The drawing under review shows one solid part. Ordinate dimensions are in mm from its lowest x, y, z. A direction names the side the tool comes from. Give positions to 0.01 mm unless a question says otherwise; leave off trailing zeros. Loops run counter-clockwise (first coordinate to the right, second up) from the corner with the lowest first, then second, coordinate; pieces in that order, holes last. Notation, with made-up numbers: M 22,20 L 78,20 A22 cw 78,55 Z; hole C 65.5,-20.5 d1. An arc over 180 degrees is marked long. Put each result on its own line as item: value. Start each with the question number.
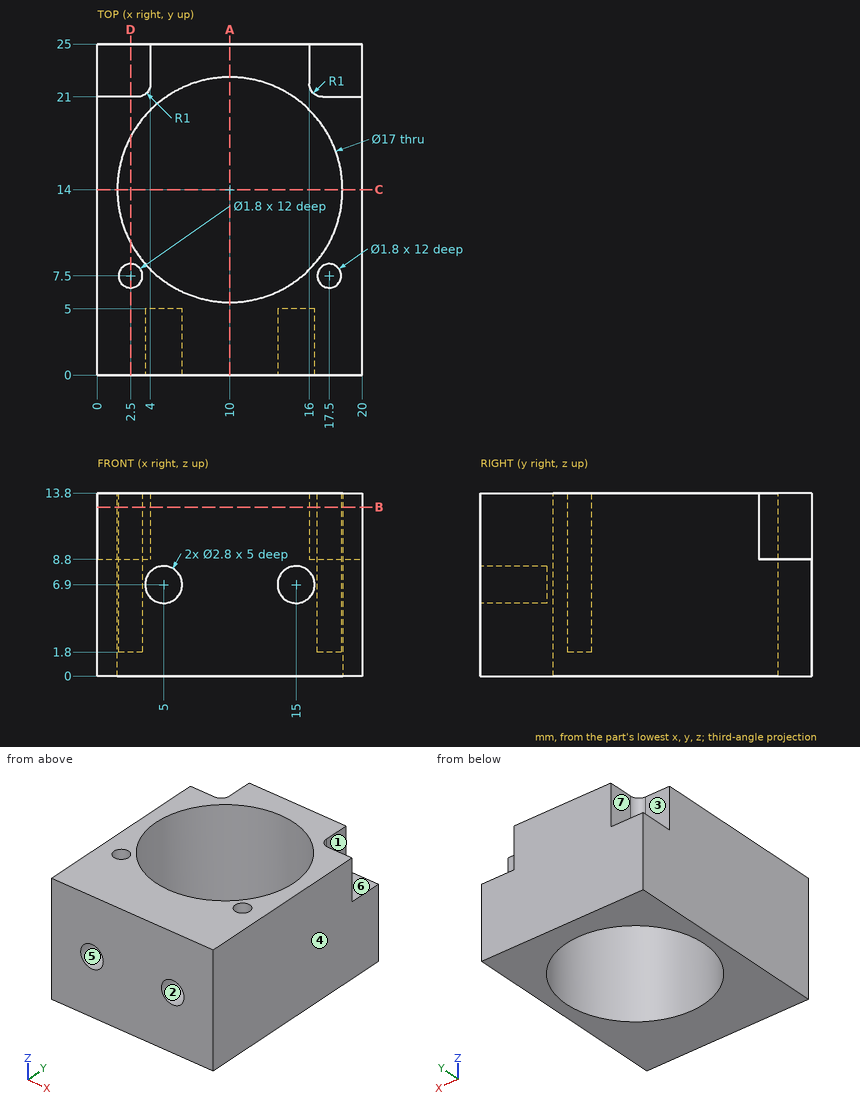
Item 1: Draft analysis for pull direction X (two halves, no side actions). For the marked faces 4, 5, 6 and 7, state which applies: +X half, -X half, draft (parallel to the pull), parting line (faces both ways), or undercut.
Item 2: Consider section A-A, the plane x = 10. Write out the cut boundary in (y, z), plus the area to 3 significant figures.
Item 3: Tool access review of the marked faces 1, 2 and 3: name each direction out of +Z, -Z, +X, -X, +Y, -Y from which nothing blocks a thin tool from reaching the whole face with its end or side.
Item 4: Consider section B-B, the plane z = 12.75. Write out the cut boundary in (x, y).
Item 5: Consider section D-D, the plane x = 2.5. Write out the cut boundary in (y, z).
Item 6: Consider section C-C, the plane y = 14. Write out the cut boundary in (x, z), plus the area to 3 significant figures.
Item 7: To check wall thickness, follow L1, parallel to Z at x = 5, y = 1.75; L2, parallel to Y at x = 17.5, z = 8.5; L3, parallel to Y at x = 2.25, z = 2.25. State the ranges of each line that lie inside material, in increasing order. Write a range as [from, to].
Item 8: Clearance check with flat-ended pins moving along their axes: pin 1 Ø6 at (x, y) = (13, 10) entering from -Z; pin 2 Ø2 at (x, y) = (2.5, 23.5) entering from +Z; pin 3 Ø2.5 at (x, z) = (2, 12.5) entering from +Y; pin 4 Ø2.5 at (y, z) = (23, 10.5) entering from -X. State where each tip first meets the part, or that it passes through.
Report:
1. face 4: +X half
1. face 5: undercut
1. face 6: draft
1. face 7: -X half
2. outline: M 0,0 L 5.5,0 L 5.5,13.8 L 0,13.8 Z; M 22.5,0 L 25,0 L 25,13.8 L 22.5,13.8 Z
2. area: 110 mm²
3. face 1: +Z, +X, +Y
3. face 2: -Y
3. face 3: +Z, -X, +Y
4. outline: M 0,0 L 20,0 L 20,21 L 17,21 A1 cw 16,22 L 16,25 L 4,25 L 4,22 A1 cw 3,21 L 0,21 Z; hole C 10,14 d17; hole C 2.5,7.5 d1.8; hole C 17.5,7.5 d1.8
5. outline: M 0,0 L 10,0 L 10,13.8 L 8.4,13.8 L 8.4,1.8 L 6.6,1.8 L 6.6,13.8 L 0,13.8 Z; M 18,0 L 25,0 L 25,8.8 L 21,8.8 L 21,13.8 L 18,13.8 Z
6. outline: M 0,0 L 1.5,0 L 1.5,13.8 L 0,13.8 Z; M 18.5,0 L 20,0 L 20,13.8 L 18.5,13.8 Z
6. area: 41.4 mm²
7. L1: [0, 5.5], [8.3, 13.8]
7. L2: [0, 6.6], [8.4, 10], [18, 25]
7. L3: [0, 6.64], [8.36, 10.51], [17.49, 25]
8. pin 1: through
8. pin 2: z = 8.8
8. pin 3: y = 21.03
8. pin 4: x = 3.97
